Work out the finished part from the listing and answer in its coordinate system (mm). A direction names the side the tool comes from. Round coordinates to 2 decimals unless told otherwise and drop trailing zeros. Write each loop counter-clockwise with the first axis right and the second up, starting at its lowest first coordinate (ties: lowest second). Pieces come first, ordered by that corner, then holes. Notation, with made-up numbers: (38.25, -32.75) - (92.25, -32.75) arc R19 ccw to (92.25, 4.25) - close; hole circle Ø2 at (66, 44.25). An arc over 180 degrees is marked (long way). Write item = value, one per line. Start each with the question number.
from build123d import *

# Parameters (mm, degrees)
SALIENTE_EXTRUIR1_DEPTH = 29.3
CROQUIS2_W              = 85.211346073
CROQUIS2_H              = 50.160748779
CORTAR_EXTRUIR1_DEPTH   = 28.35
CORTAR_EXTRUIR2_REACH   = 47.7
SALIENTE_EXTRUIR2_DEPTH = 1.15
SALIENTE_EXTRUIR3_DEPTH = 1.56
CHAFL_N1_SIZE           = 0.8
CORTAR_EXTRUIR3_DEPTH   = 30.3
CROQUIS7_R              = 9.68
SALIENTE_EXTRUIR4_DEPTH = 0.9
CROQUIS8_R              = 8.49
SALIENTE_EXTRUIR5_DEPTH = 0.83
CROQUIS9_R              = 4.445
CROQUIS9_R_2            = 1.4
SALIENTE_EXTRUIR6_DEPTH = 5.4
CHAFL_N2_SIZE           = 0.8
CORTAR_EXTRUIR4_DEPTH   = 5.4
MATRIZC1_COUNT          = 17


with BuildPart() as part:
    # Croquis1 → Saliente-Extruir1 (new body)
    with BuildSketch(Plane.XY):
        Polygon((0, 0), (59.5, 0), (59.5, 5.58), (59.355, 5.58), (59.355, 33.93), (59.5, 33.93), (59.5, 41.4), (67.34, 41.4), (67.34, 45.7), (59.5, 45.7), (59.5, 51.45), (0, 51.45), (0, 45.7), (-7.84, 45.7), (-7.84, 41.4), (0, 41.4), (0, 33.93), (0.145, 33.93), (0.145, 5.58), (0, 5.58), align=None)
    extrude(amount=SALIENTE_EXTRUIR1_DEPTH)

    # Croquis2 → Cortar-Extruir1 (cut)
    with BuildSketch(Plane(origin=(0, 5.58, 0), x_dir=(1, 0, 0), z_dir=(0, 1, 0))):
        with Locations((30.740829606, -17.065147164)):
            Rectangle(CROQUIS2_W, CROQUIS2_H)
        Polygon((0.155, -0.15), (59.345, -0.15), (59.345, -6.05), (58.685, -6.05), (58.685, -7.65), (59.345, -7.65), (59.345, -8.65), (58.685, -8.65), (58.685, -10.25), (59.345, -10.25), (59.345, -11.25), (58.685, -11.25), (58.685, -12.85), (59.345, -12.85), (59.345, -13.85), (58.685, -13.85), (58.685, -15.45), (59.345, -15.45), (59.345, -16.45), (58.685, -16.45), (58.685, -18.05), (59.345, -18.05), (59.345, -19.05), (58.685, -19.05), (58.685, -20.65), (59.345, -20.65), (59.345, -21.65), (58.685, -21.65), (58.685, -23.25), (59.345, -23.25), (59.345, -29.15), (0.155, -29.15), (0.155, -23.25), (0.815, -23.25), (0.815, -21.65), (0.155, -21.65), (0.155, -20.65), (0.815, -20.65), (0.815, -19.05), (0.155, -19.05), (0.155, -18.05), (0.815, -18.05), (0.815, -16.45), (0.155, -16.45), (0.155, -15.45), (0.815, -15.45), (0.815, -13.85), (0.155, -13.85), (0.155, -12.85), (0.815, -12.85), (0.815, -11.25), (0.155, -11.25), (0.155, -10.25), (0.815, -10.25), (0.815, -8.65), (0.155, -8.65), (0.155, -7.65), (0.815, -7.65), (0.815, -6.05), (0.155, -6.05), align=None, mode=Mode.SUBTRACT)
    extrude(amount=CORTAR_EXTRUIR1_DEPTH, mode=Mode.SUBTRACT)

    # Croquis3 → Cortar-Extruir2 (cut, up to next)
    with BuildSketch(Plane(origin=(0, 45.7, 0), x_dir=(1, 0, 0), z_dir=(0, 1, 0)), mode=Mode.PRIVATE) as cortar_extruir2_sk1:
        with BuildLine():
            Line((-8.62807943, -4.625), (-6.596389064, -4.625))
            ThreePointArc((-6.596389064, -4.625), (-1.45, -5.875), (-6.596389064, -7.125))
            Line((-6.596389064, -7.125), (-8.62807943, -7.125))
            Line((-8.62807943, -7.125), (-8.62807943, -4.625))
        make_face()
    cortar_extruir2_tool1 = extrude(cortar_extruir2_sk1.sketch, amount=-CORTAR_EXTRUIR2_REACH, mode=Mode.PRIVATE) & part.part
    add(cortar_extruir2_tool1.solids().sort_by_distance((-4.754174, 45.7, 5.875))[0], mode=Mode.SUBTRACT)
    # Croquis3 → Cortar-Extruir2 (cut, up to next)
    with BuildSketch(Plane(origin=(0, 45.7, 0), x_dir=(1, 0, 0), z_dir=(0, 1, 0)), mode=Mode.PRIVATE) as cortar_extruir2_sk2:
        with BuildLine():
            Line((68.12807943, -7.125), (66.096389064, -7.125))
            ThreePointArc((66.096389064, -7.125), (60.95, -5.875), (66.096389064, -4.625))
            Line((66.096389064, -4.625), (68.12807943, -4.625))
            Line((68.12807943, -4.625), (68.12807943, -7.125))
        make_face()
    cortar_extruir2_tool2 = extrude(cortar_extruir2_sk2.sketch, amount=-CORTAR_EXTRUIR2_REACH, mode=Mode.PRIVATE) & part.part
    add(cortar_extruir2_tool2.solids().sort_by_distance((64.254174, 45.7, 5.875))[0], mode=Mode.SUBTRACT)
    # Croquis3 → Cortar-Extruir2 (cut, up to next)
    with BuildSketch(Plane(origin=(0, 45.7, 0), x_dir=(1, 0, 0), z_dir=(0, 1, 0)), mode=Mode.PRIVATE) as cortar_extruir2_sk3:
        with BuildLine():
            Line((68.12807943, -24.675), (66.096389064, -24.675))
            ThreePointArc((66.096389064, -24.675), (60.95, -23.425), (66.096389064, -22.175))
            Line((66.096389064, -22.175), (68.12807943, -22.175))
            Line((68.12807943, -22.175), (68.12807943, -24.675))
        make_face()
    cortar_extruir2_tool3 = extrude(cortar_extruir2_sk3.sketch, amount=-CORTAR_EXTRUIR2_REACH, mode=Mode.PRIVATE) & part.part
    add(cortar_extruir2_tool3.solids().sort_by_distance((64.254174, 45.7, 23.425))[0], mode=Mode.SUBTRACT)
    # Croquis3 → Cortar-Extruir2 (cut, up to next)
    with BuildSketch(Plane(origin=(0, 45.7, 0), x_dir=(1, 0, 0), z_dir=(0, 1, 0)), mode=Mode.PRIVATE) as cortar_extruir2_sk4:
        with BuildLine():
            Line((-8.62807943, -22.175), (-6.596389064, -22.175))
            ThreePointArc((-6.596389064, -22.175), (-1.45, -23.425), (-6.596389064, -24.675))
            Line((-6.596389064, -24.675), (-8.62807943, -24.675))
            Line((-8.62807943, -24.675), (-8.62807943, -22.175))
        make_face()
    cortar_extruir2_tool4 = extrude(cortar_extruir2_sk4.sketch, amount=-CORTAR_EXTRUIR2_REACH, mode=Mode.PRIVATE) & part.part
    add(cortar_extruir2_tool4.solids().sort_by_distance((-4.754174, 45.7, 23.425))[0], mode=Mode.SUBTRACT)

    # Croquis4 → Saliente-Extruir2 (add)
    with BuildSketch(Plane(origin=(0, 51.45, 0), x_dir=(1, 0, 0), z_dir=(0, 1, 0))):
        with BuildLine():
            Line((1.15, -1.15), (44.85, -1.15))
            ThreePointArc((44.85, -1.15), (58.35, -14.65), (44.85, -28.15))
            Line((44.85, -28.15), (1.15, -28.15))
            Line((1.15, -28.15), (1.15, -1.15))
        make_face()
    extrude(amount=SALIENTE_EXTRUIR2_DEPTH)

    # Croquis5 → Saliente-Extruir3 (add)
    with BuildSketch(Plane(origin=(0, 52.6, 0), x_dir=(1, 0, 0), z_dir=(0, 1, 0))):
        with BuildLine():
            Line((8.15, -1.15), (44.85, -1.15))
            ThreePointArc((44.85, -1.15), (58.35, -14.65), (44.85, -28.15))
            Line((44.85, -28.15), (8.15, -28.15))
            Line((8.15, -28.15), (8.15, -1.15))
        make_face()
    extrude(amount=SALIENTE_EXTRUIR3_DEPTH)

    # Chaflán1
    chafl_n1_edges = [part.edges().sort_by_distance(p)[0] for p in [
        (26.5, 54.16, 1.15),
        (58.35, 54.16, 14.65),
        (26.5, 54.16, 28.15),
        (8.15, 54.16, 14.65),
    ]]
    chamfer(chafl_n1_edges, length=CHAFL_N1_SIZE)

    # Croquis6 → Cortar-Extruir3 (cut, through all)
    with BuildSketch(Plane.XY.offset(29.3)):
        Polygon((-14.418501218, 52.6), (8.15, 52.6), (21.570974014, 59.807560118), align=None)
    extrude(amount=-CORTAR_EXTRUIR3_DEPTH, mode=Mode.SUBTRACT)

    # Croquis7 → Saliente-Extruir4 (add)
    with BuildSketch(Plane(origin=(0, 54.16, 0), x_dir=(1, 0, 0), z_dir=(0, 1, 0))):
        with Locations((44.85, -14.65)):
            Circle(CROQUIS7_R)
    extrude(amount=SALIENTE_EXTRUIR4_DEPTH)

    # Croquis8 → Saliente-Extruir5 (add)
    with BuildSketch(Plane(origin=(0, 55.06, 0), x_dir=(1, 0, 0), z_dir=(0, 1, 0))):
        with Locations((44.85, -14.65)):
            Circle(CROQUIS8_R)
    extrude(amount=SALIENTE_EXTRUIR5_DEPTH)

    # Croquis9 → Saliente-Extruir6 (add)
    with BuildSketch(Plane(origin=(0, 55.89, 0), x_dir=(1, 0, 0), z_dir=(0, 1, 0))):
        with Locations((44.85, -14.65)):
            Circle(CROQUIS9_R)
        with Locations((44.85, -14.65)):
            Circle(CROQUIS9_R_2, mode=Mode.SUBTRACT)
    extrude(amount=SALIENTE_EXTRUIR6_DEPTH)

    # Chaflán2
    chafl_n2_edges = [part.edges().sort_by_distance(p)[0] for p in [
        (40.405, 61.29, 14.65),
        (43.45, 61.29, 14.65),
    ]]
    chamfer(chafl_n2_edges, length=CHAFL_N2_SIZE)

    # Croquis10 → Cortar-Extruir4 (cut)
    with BuildSketch(Plane(origin=(0, 61.29, 0), x_dir=(1, 0, 0), z_dir=(0, 1, 0))):
        Polygon((37.454169613, -6.456059857), (44.813549818, -10.705), (52.172930023, -6.456059857), align=None)
    cortar_extruir4 = extrude(amount=-CORTAR_EXTRUIR4_DEPTH, mode=Mode.SUBTRACT)

    # MatrizC1: Cortar-Extruir4 ×17 about axis
    matrizc1_axis = Axis((44.85, 0, 14.65), (0, 1, 0))
    for i in range(1, MATRIZC1_COUNT):
        add(cortar_extruir4.rotate(matrizc1_axis, i * 360 / MATRIZC1_COUNT), mode=Mode.SUBTRACT)


solid = part.part
1. Which of the six approach directions +Z, -Z, +X, -X, +Y, -Y give full straight-line access (tool end or side, diameter ignored) to faces 4 (the face through (0, 38, 14)), 5 (the face through (0.155, 20, 3)), 6 (the face through (59.5, 49, 14)), 7 (the face through (-4, 45.7, 14))?
2. Find section B-B on x = 37.5. Give the vertices of the cut face in (y, z).
3. Find section A-A on x = 25. Give the vertices of the cut face in (y, z).
4. Each of these flat-tipped pins is pushed along its axis until it touches: pin 1 (0.8 mm diameter, centred on y = 16, z = 7, fed in from -X) (3 decimals); pin 2 (1.8 mm diameter, centred on y = 22.5, z = 14.5, fed in from +X) (3 decimals); pin 3 (22.5 mm diameter, centred on x = 24, y = 22.5, fed in from +Z); pin 4 (5 mm diameter, centred on x = -4.175, z = 5.875, fed in from -Y). Where does it stop, or does it pass through?
5. For a pull along X with two mould halves and no side action, classify faces 1 (the face through (45, 55.89, 15)), 2 (the face through (9.58, 53.37, 14.84)), 3 (the face through (59.345, 20, 26)) as released by +X, released by -X, zero draft, split by the parting line, or undercut.
6. Consider line 1 (Y direction, x = 45, z = 7.75); line 2 (X direction, y = 33.5, z = 21.5) (3 decimals); line 3 (X direction, y = 47, z = 9.25). Determine where each line is inside the solid, lowest interval first.
Answer key:
q1.face_4 = +Z, -Z, -X, -Y
q1.face_5 = +Z, -Z, -X
q1.face_6 = +Z, -Z, +X, +Y
q1.face_7 = +Z, -Z, -X, +Y
q2.outline = (0, 0) - (5.58, 0) - (5.58, 0.15) - (33.93, 0.15) - (33.93, 0) - (51.45, 0) - (51.45, 1.15) - (53.36, 1.15) - (54.16, 1.95) - (54.16, 8.35) - (55.06, 8.35) - (55.06, 10.4) - (55.89, 10.4) - (55.89, 18.9) - (55.06, 18.9) - (55.06, 20.95) - (54.16, 20.95) - (54.16, 27.35) - (53.36, 28.15) - (51.45, 28.15) - (51.45, 29.3) - (33.93, 29.3) - (33.93, 29.15) - (5.58, 29.15) - (5.58, 29.3) - (0, 29.3) - close
q3.outline = (0, 0) - (5.58, 0) - (5.58, 0.15) - (33.93, 0.15) - (33.93, 0) - (51.45, 0) - (51.45, 1.15) - (53.36, 1.15) - (54.16, 1.95) - (54.16, 27.35) - (53.36, 28.15) - (51.45, 28.15) - (51.45, 29.3) - (33.93, 29.3) - (33.93, 29.15) - (5.58, 29.15) - (5.58, 29.3) - (0, 29.3) - close
q4.pin_1 = 0.815
q4.pin_2 = 59.345
q4.pin_3 = 29.15
q4.pin_4 = through
q5.face_1 = undercut
q5.face_2 = released by -X
q5.face_3 = released by +X
q6.line_1 = 0 to 55.89
q6.line_2 = 0.155 to 59.345
q6.line_3 = 0 to 59.5
